Drawing for the job (mm, zero at the part's lowest x, y, z). Coordinates: 2 decimals unless noted, no trailing zeros. Write each loop counter-clockwise with the first axis right and the second up, starting at its lowest first coordinate (ties: lowest second). Pieces come first, ordered by that corner, then holes. Notation, with made-up numbers: M -29,4 L 22,4 A12 ccw 22,22 Z; hole C 57.25,20.25 d7. An arc over 180 degrees is marked long. Use a Markdown table: item, result. Add a question column.
Q1. Slice it at C-C on z = 54.5. Write the cut outline in (x, y), then the cut area to 3 significant figures.
Q2. Pin check, flat tips, straight feed: pin 1 Ø4 at (y, z) = (5, 14.5) entering from +X; pin 2 Ø4 at (x, z) = (5, 47) entering from +Y; pin 3 Ø1.5 at (y, z) = (6.5, 11.5) entering from -X. Stop position of each tip, or through.
Q3. Mould opens along Z. For the marked faces 1, 2 and 3 say: released by +Z, released by -Z, zero draft, split by the parting line, or undercut.
Q4. Slice it at A-A on y = 3.5. Write the cut outline in (x, z).
Q5. Wall check: L1, parallel to Z at x = 2, y = 6.5; L2, parallel to Y at x = 3.5, z = 43; L3, parallel to Y at x = 1.25, z = 54.5. Give the ranges that are in metal, low to high. Write a range as from..to.
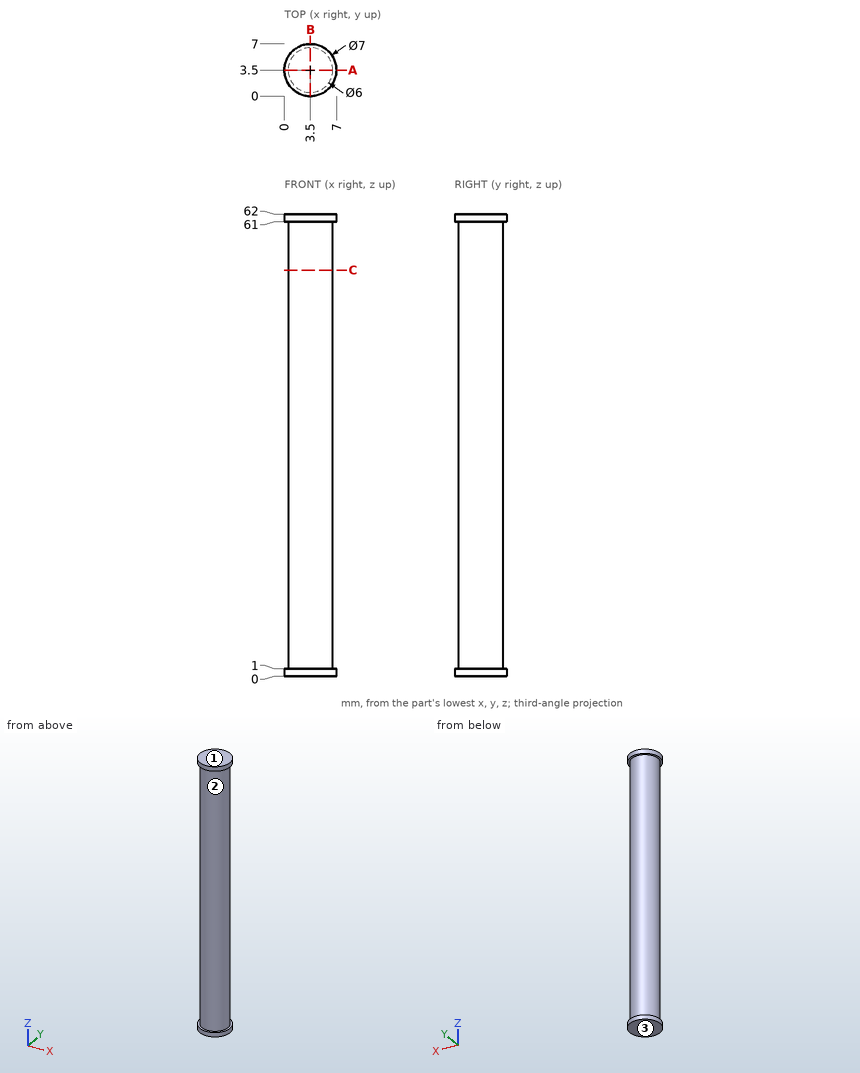
Recorded:
| question | item | result |
|---|---|---|
| 1 | outline | C 3.5,3.5 d6 |
| 1 | area | 28.3 mm² |
| 2 | pin 1 | x = 6.5 |
| 2 | pin 2 | y = 6.5 |
| 2 | pin 3 | x = 1.52 |
| 3 | face 1 | released by +Z |
| 3 | face 2 | undercut |
| 3 | face 3 | released by -Z |
| 4 | outline | M 0,0 L 7,0 L 7,1 L 6.5,1 L 6.5,61 L 7,61 L 7,62 L 0,62 L 0,61 L 0.5,61 L 0.5,1 L 0,1 Z |
| 5 | L1 | 0..1, 61..62 |
| 5 | L2 | 0.5..6.5 |
| 5 | L3 | 1.52..5.48 |
